```python
from build123d import *

# Parameters (mm, degrees)
F0_W          = 138
F0_H          = 28.5
F1_DEPTH      = 3.8
F2_W          = 28.5
F2_H          = 28.5
F3_DEPTH      = 3.28
F3_DEPTH_BACK = 6.56
F5_R          = 1.3
F6_DEPTH      = 9.84
F7_DEPTH      = 3.8


with BuildPart() as f1:
    # F0 (on Front) → F1 (new body)
    with BuildSketch(Plane.XZ):
        with Locations((69, 14.25)):
            Rectangle(F0_W, F0_H)
    extrude(amount=F1_DEPTH)

    # F2 (on face) → F3 (join, two sides)
    with BuildSketch(Plane.XZ.offset(3.8)) as f3_sk:
        with Locations((123.75, 14.25)):
            Rectangle(F2_W, F2_H)
    extrude(amount=F3_DEPTH)
    extrude(f3_sk.sketch, amount=-F3_DEPTH_BACK)

    # F5 (on face) → F6 (cut, through all)
    with BuildSketch(Plane.XZ.offset(7.08)):
        with Locations((125, 14.25)):
            Circle(F5_R)
    extrude(amount=-F6_DEPTH, mode=Mode.SUBTRACT)

    # F4 (on face) → F7 (cut, through all)
    with BuildSketch(Plane.XZ.offset(3.8)):
        with BuildLine():
            ThreePointArc((24.68, 16.25), (23.265786, 15.664214), (22.68, 14.25))
            Line((22.68, 14.25), (41.68, 14.25))
            ThreePointArc((41.68, 14.25), (41.094214, 15.664214), (39.68, 16.25))
            Line((39.68, 16.25), (24.68, 16.25))
        make_face()
        with BuildLine():
            ThreePointArc((60.68, 16.25), (59.265786, 15.664214), (58.68, 14.25))
            Line((58.68, 14.25), (77.68, 14.25))
            ThreePointArc((77.68, 14.25), (77.094214, 15.664214), (75.68, 16.25))
            Line((75.68, 16.25), (60.68, 16.25))
        make_face()
        with BuildLine():
            Line((77.68, 14.25), (58.68, 14.25))
            ThreePointArc((58.68, 14.25), (59.265786, 12.835786), (60.68, 12.25))
            Line((60.68, 12.25), (75.68, 12.25))
            ThreePointArc((75.68, 12.25), (77.094214, 12.835786), (77.68, 14.25))
        make_face()
        with BuildLine():
            Line((41.68, 14.25), (22.68, 14.25))
            ThreePointArc((22.68, 14.25), (23.265786, 12.835786), (24.68, 12.25))
            Line((24.68, 12.25), (39.68, 12.25))
            ThreePointArc((39.68, 12.25), (41.094214, 12.835786), (41.68, 14.25))
        make_face()
    extrude(amount=-F7_DEPTH, mode=Mode.SUBTRACT)


solid = f1.part
```
Geometry check sheet. Reference: the model listing, model coordinates, mm. A direction names the side the tool comes from. Round coordinates to 2 decimals unless told otherwise and drop trailing zeros. Order: outer loops, then holes, each group sorted by start corner. A loop starts at its lowest first (then second) coordinate and runs counter-clockwise, first axis right, second up. Notation, with made-up numbers: (-28, 82.5) - (-13, 82.5) arc R34 cw to (-13, 112.5) - close; hole circle Ø10 at (48.5, 39.5). An arc over 180 degrees is marked (long way). Use a Markdown table: item, result. Add a question column.
1) Section check B-B (y = -1.5). Record the cut outline in (x, z), then the cut area to 3 significant figures.
2) Section check C-C (z = 26.75). Record the cut outline in (x, y), then the cut area to 3 significant figures.
3) Thickness scan on line 1 along X through (y, z) = (-2.75, 14); line 2 along Z through (x, y) = (66.5, -2.75); line 3 along Z through (x, y) = (125, -0.25). Record the ranges inside material, lowest first.
4) Mould release check, pull along X, two halves, no side actions. Record for faces 1 (the flat face through (109.5, 1, 14)), 2 (the cylindrical face through (126.2, -2.23, 13.75)), 3 (the flat face through (54, -3.8, 14)): released by +X, released by -X, zero draft, split by the parting line, or undercut.
5) Section check D-D (x = 47.5). Record the cut outline in (y, z).
6) Set-up check for faces 4 (the flat face through (109.5, -5, 14)), 5 (the flat face through (54, 0, 14)), 6 (the flat face through (68, -2, 16.25)): record each of +Z, -Z, +X, -X, +Y, -Y from which the full face is reachable in a straight line by a thin tool's end or side.
7) Gauge pin test, flat ends, axial feed: P1, Ø8, axis at x = 36.5, z = 3, coming from the -Y side; P2, Ø0.8, axis at y = 1.5, z = 9, coming from the -X side. Record the tip position at first contact, or that the pin passes through.
8) Section check A-A (x = 125). Record the cut outline in (y, z), then the cut area to 3 significant figures.
Established:
| question | item | result |
|---|---|---|
| 1 | outline | (0, 0) - (138, 0) - (138, 28.5) - (0, 28.5) - close; hole (22.68, 14.25) arc R2 ccw to (24.68, 12.25) - (39.68, 12.25) arc R2 ccw to (41.68, 14.25) arc R2 ccw to (39.68, 16.25) - (24.68, 16.25) arc R2 ccw to start; hole (58.68, 14.25) arc R2 ccw to (60.68, 12.25) - (75.68, 12.25) arc R2 ccw to (77.68, 14.25) arc R2 ccw to (75.68, 16.25) - (60.68, 16.25) arc R2 ccw to start; hole circle Ø2.6 at (125, 14.25) |
| 1 | area | 3,780 mm2 |
| 2 | outline | (0, -3.8) - (109.5, -3.8) - (109.5, -7.08) - (138, -7.08) - (138, 2.76) - (109.5, 2.76) - (109.5, 0) - (0, 0) - close |
| 2 | area | 697 mm2 |
| 3 | line 1 | 0 to 22.7, 41.66 to 58.7, 77.66 to 123.72, 126.28 to 138 |
| 3 | line 2 | 0 to 12.25, 16.25 to 28.5 |
| 3 | line 3 | 0 to 12.95, 15.55 to 28.5 |
| 4 | face 1 | released by -X |
| 4 | face 2 | undercut |
| 4 | face 3 | zero draft |
| 5 | outline | (-3.8, 0) - (0, 0) - (0, 28.5) - (-3.8, 28.5) - close |
| 6 | face 4 | +Z, -Z, -X, -Y |
| 6 | face 5 | +Z, -Z, -X, +Y |
| 6 | face 6 | +Y, -Y |
| 7 | P1 | y = -3.8 |
| 7 | P2 | x = 109.5 |
| 8 | outline | (-7.08, 0) - (2.76, 0) - (2.76, 12.95) - (-7.08, 12.95) - close; (-7.08, 15.55) - (2.76, 15.55) - (2.76, 28.5) - (-7.08, 28.5) - close |
| 8 | area | 255 mm2 |
